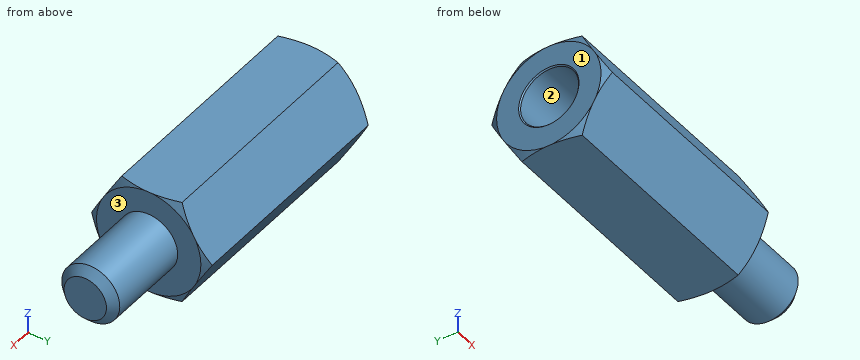
from build123d import *

# Parameters (mm, degrees)
SKETCH2_R         = 1.25
EXTRUDE1_DEPTH    = 3.9
CHAMFER1_SIZE     = 0.3375
EXTRUDE4_DEPTH    = 10
SKETCH8_OUTSIDE_W = 62.666
SKETCH8_OUTSIDE_H = 63.362
SKETCH8_OUTSIDE_R = 2.25
EXTRUDE5_DEPTH    = 15.318606776
EXTRUDE5_DRAFT    = -60
SKETCH9_OUTSIDE_W = 49.696
SKETCH9_OUTSIDE_H = 50.392
SKETCH9_OUTSIDE_R = 2.25
EXTRUDE6_DEPTH    = 11.574142991
EXTRUDE6_DRAFT    = -60
EXTRUDE7_START    = -4.8
SKETCH10_R        = 1.25
EXTRUDE7_DEPTH    = 4.8
SKETCH13_R        = 1.3008
EXTRUDE8_DEPTH    = 15.318606776


with BuildPart() as part:
    # Sketch2 → Extrude1 (new body)
    with BuildSketch(Plane(origin=(6.95, 0, 0), x_dir=(0, 0, -1), z_dir=(1, 0, 0))):
        Circle(SKETCH2_R)
    extrude(amount=-EXTRUDE1_DEPTH)

    # Chamfer1
    chamfer1_edges = [part.edges().sort_by_distance(p)[0] for p in [
        (6.95, 0, 1.25),
    ]]
    chamfer(chamfer1_edges, length=CHAMFER1_SIZE)

    # Sketch7 → Extrude4 (add)
    with BuildSketch(Plane(origin=(3.05, 0, 0), x_dir=(0, 0, -1), z_dir=(1, 0, 0))):
        Polygon((0, 2.598076211), (-2.25, 1.299038106), (-2.25, -1.299038106), (0, -2.598076211), (2.25, -1.299038106), (2.25, 1.299038106), align=None)
    extrude(amount=-EXTRUDE4_DEPTH)


with BuildPart() as extrude5_tool:
    # Sketch8 outside → Extrude5 (with draft: the straight prism first)
    with BuildSketch(Plane.ZY.offset(6.95)):
        Rectangle(SKETCH8_OUTSIDE_W, SKETCH8_OUTSIDE_H)
        Circle(SKETCH8_OUTSIDE_R, mode=Mode.SUBTRACT)
    extrude(amount=-EXTRUDE5_DEPTH)
    # Extrude5: the draft: its side faces are tilted about the plane it starts from
    extrude5_sides = [extrude5_tool.faces().sort_by_distance(p)[0] for p in [
        (0.709303388, -31.681, 0),
        (0.709303388, 0, 31.333),
        (0.709303388, 31.681, 0),
        (0.709303388, 0, -31.333),
        (0.709303388, 0, -2.25),
    ]]
    draft(extrude5_sides, Plane.ZY.offset(6.95), EXTRUDE5_DRAFT)


with BuildPart() as part_1:
    add(part.part)

    # Extrude5: cut by extrude5_tool
    add(extrude5_tool.part, mode=Mode.SUBTRACT)


with BuildPart() as extrude6_tool:
    # Sketch9 outside → Extrude6 (with draft: the straight prism first)
    with BuildSketch(Plane(origin=(3.05, 0, 0), x_dir=(0, 0, -1), z_dir=(1, 0, 0))):
        Rectangle(SKETCH9_OUTSIDE_W, SKETCH9_OUTSIDE_H)
        Circle(SKETCH9_OUTSIDE_R, mode=Mode.SUBTRACT)
    extrude(amount=-EXTRUDE6_DEPTH)
    # Extrude6: the draft: its side faces are tilted about the plane it starts from
    extrude6_sides = [extrude6_tool.faces().sort_by_distance(p)[0] for p in [
        (-2.737071496, -25.196, 0),
        (-2.737071496, 0, -24.848),
        (-2.737071496, 25.196, 0),
        (-2.737071496, 0, 24.848),
        (-2.737071496, 0, 2.25),
    ]]
    draft(extrude6_sides, Plane(origin=(3.05, 0, 0), x_dir=(0, 0, -1), z_dir=(1, 0, 0)), EXTRUDE6_DRAFT)


with BuildPart() as part_2:
    add(part_1.part)

    # Extrude6: cut by extrude6_tool
    add(extrude6_tool.part, mode=Mode.SUBTRACT)

    # Sketch10 → Extrude7 (cut)
    with BuildSketch(Plane.ZY.offset(6.95).offset(EXTRUDE7_START)):
        with Locations(Location((0, 0, 0), (0, 0, 180))):
            Circle(SKETCH10_R)
    extrude(amount=EXTRUDE7_DEPTH, mode=Mode.SUBTRACT)

    # Sketch13 → Extrude8 (cut)
    with BuildSketch(Plane.ZY.offset(6.95)):
        Circle(SKETCH13_R)
    extrude(amount=EXTRUDE8_DEPTH, mode=Mode.SUBTRACT)

    # Extrude8 cone 1 section (through the dimple's axis) → Extrude8 other way (revolve, cut)
    with BuildSketch(Plane(origin=(-6.95, 0, 0), x_dir=(0, 0, 1), z_dir=(0, 1, 0))):
        Polygon((0, 0), (1.3008, 0), (0, 1.3008), align=None)
    revolve(axis=Axis((-6.95, 0, 0), (1, 0, 0)), mode=Mode.SUBTRACT)


solid = part_2.part
Work out the finished part from the listing and answer in its coordinate system (mm). Face numbers are marked on the shaded views. A direction names the side the tool comes from. Give positions to 0.01 mm unless a question says otherwise; leave off trailing zeros. Write each loop counter-clockwise with the first axis right and the second up, starting at its lowest first coordinate (ties: lowest second). Pieces come first, ordered by that corner, then holes.
Q1. The part is cut by section A-A on x = -4. Give the vertices of the cut face in (y, z).
Answer:
outline: (-2.6, 0) - (-1.3, -2.25) - (1.3, -2.25) - (2.6, 0) - (1.3, 2.25) - (-1.3, 2.25) - close; hole circle Ø2.5 at (0, 0)
Q2. Given pin 1 (1 mm diameter, centred on x = -3, z = -1, fed in from +Y), flat-ended and moving along its own axis, determine where the tip first touches the part or whether it passes through.
Answer:
pin 1: stops at y = 2.31
Q3. Straight lines are drawn through the part: L1, parallel to X at y = 0.8, z = 1.3; L2, parallel to Z at x = -2.25, y = 0.85. For each, find the intervals that lie inside material, in ascending order.
Answer:
L1: x = -6.95 to 3.05
L2: z = -2.25 to -0.92, 0.92 to 2.25
Q4. The part is cut by section B-B on x = 2. Give the vertices of the cut face in (y, z), and give its area (3 significant figures).
Answer:
outline: (-2.6, 0) - (-1.3, -2.25) - (1.3, -2.25) - (2.6, 0) - (1.3, 2.25) - (-1.3, 2.25) - close
area: 17.5 mm2
Q5. The part is cut by section C-C on x = 6.25. Give the vertices of the cut face in (y, z), and give its area (3 significant figures).
Answer:
outline: circle Ø2.5 at (0, 0)
area: 4.91 mm2
Q6. A tool of negligible diameter and unlimited length cuts with its end or side. For the marked faces 1, 2 and 3, from which of +Z, -Z, +X, -X, +Y, -Y can it reach the whole face along a straight path? Write none if from no direction.
Answer:
face 1: +Z, -Z, -X, +Y, -Y
face 2: -X
face 3: +X
